from build123d import *

# Parameters (mm, degrees)
SKETCH1_W           = 120
SKETCH1_H           = 120
BOSS_EXTRUDE1_DEPTH = 5
SKETCH2_W           = 100
SKETCH2_H           = 100
SKETCH2_W_2         = 80
SKETCH2_H_2         = 80
EXTRUDE_THIN1_DEPTH = 1620
FILLET1_R           = 10
SKETCH4_W           = 28.971165854
SKETCH4_H           = 139.886747586
CUT_EXTRUDE1_DEPTH  = 1631.529055246
SKETCH5_R           = 40
CUT_EXTRUDE2_DEPTH  = 1629.841612926


with BuildPart() as part:
    # Sketch1 → Boss-Extrude1 (new body)
    with BuildSketch(Plane.XY):
        Rectangle(SKETCH1_W, SKETCH1_H)
    extrude(amount=BOSS_EXTRUDE1_DEPTH)

    # Sketch2 → Extrude-Thin1 (add)
    with BuildSketch(Plane.XY.offset(5)):
        Rectangle(SKETCH2_W, SKETCH2_H)
        Rectangle(SKETCH2_W_2, SKETCH2_H_2, mode=Mode.SUBTRACT)
    extrude(amount=EXTRUDE_THIN1_DEPTH)

    # Fillet1
    fillet1_edges = [part.edges().sort_by_distance(p)[0] for p in [
        (50, -50, 815),
        (50, 50, 815),
        (-50, 50, 815),
        (-50, -50, 815),
    ]]
    fillet(fillet1_edges, radius=FILLET1_R)

    # Sketch4 → Cut-Extrude1 (cut, through all)
    with BuildSketch(Plane(origin=(60, 0, 0), x_dir=(0, 0, -1), z_dir=(1, 0, 0))):
        with Locations((9.485582927, 4.056648122)):
            Rectangle(SKETCH4_W, SKETCH4_H)
    extrude(amount=-CUT_EXTRUDE1_DEPTH, mode=Mode.SUBTRACT)

    # Sketch5 → Cut-Extrude2 (cut, through all)
    with BuildSketch(Plane(origin=(50, 0, 0), x_dir=(0, 0, -1), z_dir=(1, 0, 0))):
        with Locations(Location((-815, 0, 0), (0, 0, 270))):
            Circle(SKETCH5_R)
    extrude(amount=-CUT_EXTRUDE2_DEPTH, mode=Mode.SUBTRACT)


solid = part.part
Check sheet for the modelled part. Datum: model origin and axes. Units: mm. A direction names the side the tool comes from. Round coordinates to 2 decimals unless told otherwise and drop trailing zeros. Order: outer loops, then holes, each group sorted by start corner. A loop starts at its lowest first (then second) coordinate and runs counter-clockwise, first axis right, second up.
(1) Draft check along Z on faces 1 (the cylindrical face through (45.07, 8.67, 854.05)), 2 (the flat face through (50, -1, 404)), 3 (the flat face through (-45, 1, 1625)). Enter one of: pulls with the +Z half, pulls with the -Z half, needs draft (parallel to the pull), parting line crosses it, or undercut.
(2) Access from +Z, -Z, +X, -X, +Y, -Y to the whole of each face (thin tool, end or side, straight path). Record for faces 4 (the flat face through (40, -1, 404)), 5 (the flat face through (-50, -1, 404)).
(3) Scan lines: probe 1 along X at (y, z) = (-13.5, 1361.5); probe 2 along Y at (x, z) = (42, 815). Record each from-to range of solid material in increasing order.
(4) Cross-section at C-C, the plane z = 653. Enter the section's corners in (x, y).
(5) Cross-section at B-B, the plane x = -20. Enter the section's corners in (y, z).
(6) Cross-section at A-A, the plane y = 0. Enter the section's corners in (x, z), and give its area (3 significant figures).
Check sheet entries:
1. face 1: undercut
1. face 2: needs draft
1. face 3: pulls with the +Z half
2. face 4: +Z, -Z
2. face 5: +Z, -Z, -X, +Y, -Y
3. probe 1: x = -50 to -40, 40 to 50
3. probe 2: y = -49.8 to -40, 40 to 49.8
4. outline: (-50, -40) arc R10 ccw to (-40, -50) - (40, -50) arc R10 ccw to (50, -40) - (50, 40) arc R10 ccw to (40, 50) - (-40, 50) arc R10 ccw to (-50, 40) - close; hole (-40, -40) - (40, -40) - (40, 40) - (-40, 40) - close
5. outline: (-50, 5) - (-40, 5) - (-40, 1625) - (-50, 1625) - close; (40, 5) - (50, 5) - (50, 1625) - (40, 1625) - close
6. outline: (-50, 5) - (-40, 5) - (-40, 775) - (-50, 775) - close; (-50, 855) - (-40, 855) - (-40, 1625) - (-50, 1625) - close; (40, 5) - (50, 5) - (50, 775) - (40, 775) - close; (40, 855) - (50, 855) - (50, 1625) - (40, 1625) - close
6. area: 30,800 mm2
